Design review of the part shown in the three views and the two pictorial views. Dimensions are in mm from the part's minimum x, y and z. Coordinates: 2 decimals unless noted, no trailing zeros. Loops run counter-clockwise (first coordinate to the right, second up) from the corner with the lowest first, then second, coordinate; pieces in that order, holes last. Notation, with made-up numbers: (18, 68) - (75, 68) arc R33 cw to (75, 102) - close; hole circle Ø10 at (49, 1.5). An arc over 180 degrees is marked (long way). One line per item, written item: value. Start each with the question number.
1. Take a section at B-B, the plane z = 23. State the section outline as (x, y) points, and give its area (3 significant figures).
2. To check wall thickness, follow line 1 (X direction, y = 132.5, z = 15.75); line 2 (Z direction, x = 7, y = 116); line 3 (X direction, y = 95, z = 4). State the ranges of each line that lie inside material, in increasing order. Write a range as from..to.
3. Insertion check: pin 1 (1.5 mm diameter, centred on y = 122, z = 20.5, fed in from -X); pin 2 (4 mm diameter, centred on y = 66.5, z = 6.5, fed in from +X). Each pin has a flat end and moves straight along its axis. Give the tip position at first contact, or say it passes through.
4. Take a section at C-C, the plane x = 6.5. State the section outline as (y, z) points.
5. Take a section at A-A, the plane y = 72. State the section outline as (x, z) points.
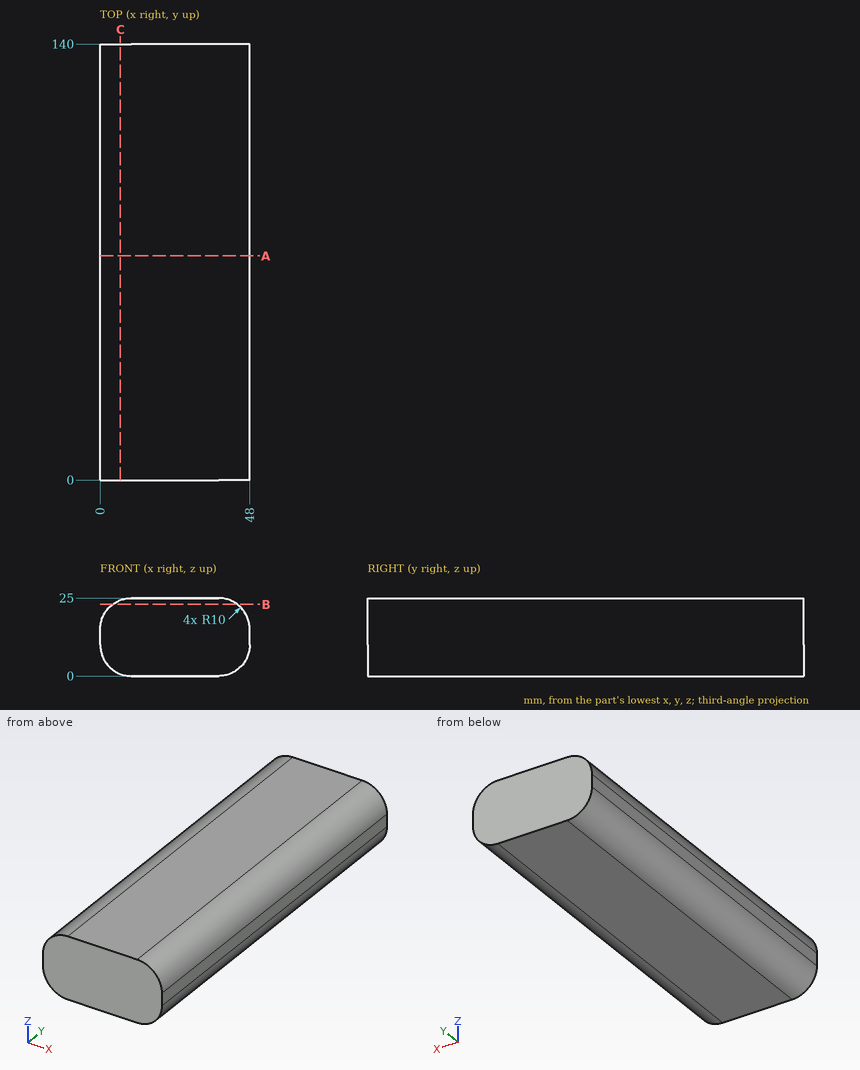
Solutions:
1. outline: (4, 0) - (44, 0) - (44, 140) - (4, 140) - close
1. area: 5,600 mm2
2. line 1: 0.03..47.97
2. line 2: 0.46..24.54
2. line 3: 2..46
3. pin 1: x = 1.2
3. pin 2: x = 47.89
4. outline: (0, 0.63) - (140, 0.63) - (140, 24.37) - (0, 24.37) - close
5. outline: (0, 10) arc R10 ccw to (10, 0) - (38, 0) arc R10 ccw to (48, 10) - (48, 15) arc R10 ccw to (38, 25) - (10, 25) arc R10 ccw to (0, 15) - close
